Geometry: final body of the model. Coordinates: model frame, mm. Coordinates: 2 decimals unless noted, no trailing zeros. Write each loop counter-clockwise with the first axis right and the second up, starting at its lowest first coordinate (ties: lowest second). Pieces come first, ordered by that corner, then holes.
from build123d import *

# Parameters (mm, degrees)
F0_R     = 3.2512
F0_R_2   = 2.413
F1_DEPTH = 0.889


with BuildPart() as f1:
    # F0 (on Front) → F1 (new body)
    with BuildSketch(Plane.XZ):
        with BuildLine():
            ThreePointArc((-34.7836, 56.482241), (-35.681625, 56.110266), (-36.0536, 55.212241))
            Line((-36.0536, 55.212241), (-36.0536, -55.023759))
            ThreePointArc((-36.0536, -55.023759), (-35.681625, -55.921785), (-34.7836, -56.293759))
            Line((-34.7836, -56.293759), (35.8284, -56.293759))
            ThreePointArc((35.8284, -56.293759), (36.726426, -55.921785), (37.0984, -55.023759))
            Line((37.0984, -55.023759), (37.0984, 55.212241))
            ThreePointArc((37.0984, 55.212241), (36.726426, 56.110266), (35.8284, 56.482241))
            Line((35.8284, 56.482241), (24.3984, 56.482241))
            Line((24.3984, 56.482241), (24.3984, -38.513759))
            Line((24.3984, -38.513759), (10.1744, -38.513759))
            Line((10.1744, -38.513759), (10.1744, -22.511759))
            Line((10.1744, -22.511759), (-9.1296, -22.511759))
            Line((-9.1296, -22.511759), (-9.1296, -38.513759))
            Line((-9.1296, -38.513759), (-23.3536, -38.513759))
            Line((-23.3536, -38.513759), (-23.3536, 56.482241))
            Line((-23.3536, 56.482241), (-34.7836, 56.482241))
        make_face()
        with Locations((-30.022221, -48.062544)):
            Circle(F0_R, mode=Mode.SUBTRACT)
        with Locations((-16.222711, -48.062544)):
            Circle(F0_R, mode=Mode.SUBTRACT)
        with Locations((-4.467035, -30.334959)):
            Circle(F0_R, mode=Mode.SUBTRACT)
        with Locations((-30.022221, -26.952723)):
            Circle(F0_R, mode=Mode.SUBTRACT)
        with Locations((-30.022221, -5.842898)):
            Circle(F0_R, mode=Mode.SUBTRACT)
        with Locations((17.563765, -48.062544)):
            Circle(F0_R, mode=Mode.SUBTRACT)
        with Locations((5.348405, -30.334959)):
            Circle(F0_R, mode=Mode.SUBTRACT)
        with Locations((30.7484, -48.062544)):
            Circle(F0_R, mode=Mode.SUBTRACT)
        with Locations((30.7484, -26.952723)):
            Circle(F0_R, mode=Mode.SUBTRACT)
        with Locations((30.7484, -5.842898)):
            Circle(F0_R, mode=Mode.SUBTRACT)
        with Locations((-30.022221, 13.207102)):
            Circle(F0_R, mode=Mode.SUBTRACT)
        with Locations((-30.022221, 23.386041)):
            Circle(F0_R_2, mode=Mode.SUBTRACT)
        with Locations((-30.022221, 44.671241)):
            Circle(F0_R, mode=Mode.SUBTRACT)
        with Locations((-30.022221, 51.910241)):
            Circle(F0_R_2, mode=Mode.SUBTRACT)
        with Locations((30.7484, 13.207102)):
            Circle(F0_R, mode=Mode.SUBTRACT)
        with Locations((30.7484, 23.386041)):
            Circle(F0_R_2, mode=Mode.SUBTRACT)
        with Locations((30.7484, 44.671241)):
            Circle(F0_R, mode=Mode.SUBTRACT)
        with Locations((30.7484, 51.910241)):
            Circle(F0_R_2, mode=Mode.SUBTRACT)
    extrude(amount=F1_DEPTH)


solid = f1.part
Item 1: Pin query (flat end, axial travel): pin 1 (8.5 mm diameter, centred on x = -30.02, z = -48.06, fed in from -Y); pin 2 (3 mm diameter, centred on x = -30.02, z = 23.39, fed in from +Y). Return the tip coordinate at first contact, or that it passes through.
Derived:
pin 1: stops at y = -0.89
pin 2: passes through
Item 2: Pull-direction query (Z, two-part tool) for faces 1 (the cylindrical face through (-2.97, -0.44, -33.22)), 2 (the flat face through (-8, -0.889, -24)); classes: released by +Z, released by -Z, zero draft, split by the parting line, or undercut.
Derived:
face 1: undercut
face 2: zero draft
Item 3: Section A-A, the plane x = -30.5. State how many separate pieces and enclosed holes the cut face has, plus the area to 3 significant figures.
Derived:
separate pieces: 8
enclosed holes: 0
area: 63.3 mm2
Item 4: Section D-D, the plane x = -18. Output: boundary loops of the cut face in (y, z), plus the area to 3 significant figures.
Derived:
outline: (-0.89, -56.29) - (0, -56.29) - (0, -50.78) - (-0.89, -50.78) - close; (-0.89, -45.34) - (0, -45.34) - (0, -38.51) - (-0.89, -38.51) - close
area: 11.0 mm2
Item 5: Section B-B, the plane z = -12. Output: boundary loops of the cut face in (x, y).
Derived:
outline: (-36.05, -0.89) - (-23.35, -0.89) - (-23.35, 0) - (-36.05, 0) - close; (24.4, -0.89) - (37.1, -0.89) - (37.1, 0) - (24.4, 0) - close
Item 6: Material intervals for probe 1 along X at (y, z) = (-0.55, -34.5); probe 2 along X at (y, z) = (-0.1, 6.5); probe 3 along Z at (x, y) = (17.5, -0.4), sorted ascending.
Derived:
probe 1: x = -36.05 to -23.35, -9.13 to 10.17, 24.4 to 37.1
probe 2: x = -36.05 to -23.35, 24.4 to 37.1
probe 3: z = -56.29 to -51.31, -44.81 to -38.51
